Can you work these out from the model? Positions are in its coordinate system, mm. A direction names the side the tool comes from. Coordinates: 2 decimals unless noted, no trailing zeros. Loops run counter-clockwise (first coordinate to the right, second up) from the corner with the lowest first, then second, coordinate; pieces in that order, holes last. Notation, with made-up numbers: (75, 69) -> (94, 69) arc R8 cw to (94, 77) -> close; hole circle Ø5 at (-34.5, 65.25). An arc over 180 degrees is marked (long way). Use one line per item in the form item = value. Start each with the question number.
(1) I'm going to push flat-ended pins straight in: pin 1 (4 mm diameter, centred on x = -1, z = -2, fed in from -Y); pin 2 (3 mm diameter, centred on y = -8, z = -2.5, fed in from -X); pin 3 (6 mm diameter, centred on y = 2.5, z = 4, fed in from +X). Where does each tip first touch, or does it pass through?
(2) Imagine slicing it at B-B (x = 0). List the corners of the cut face in (y, z) for me, plus the area to 3 significant figures.
(3) I need wall thicknesses on line 1 (Y direction, x = -2.25, z = 3.25); line 2 (Z direction, x = 2, y = -13.5); line 3 (Z direction, x = -5, y = -8). Which ranges of each line are inside material? Lowest first, please. Write a range as [from, to].
(4) On a 3-axis mill with a long thin cutter (end or side, diameter ignored), from which of +Z, -Z, +X, -X, +Y, -Y can I reach the whole of each face in a straight line? I mean faces 1 (the conical face through (5.365, -8.619, 2.79)), 2 (the cylindrical face through (3.71, 3.45, 4.84)), 3 (the flat face through (0, 7, 0)). Say none if no direction works.
(5) Imagine slicing it at C-C (z = 0). List the corners of the cut face in (x, y) for me, plus the area to 3 significant figures.
(6) Imagine slicing it at A-A (y = -23). List the corners of the cut face in (x, z) for me.
```python
from build123d import *

# Parameters (mm, degrees)
SKETCH2_R           = 6.1
BOSS_EXTRUDE1_DEPTH = 7
SKETCH3_R           = 0.35
BOSS_EXTRUDE2_DEPTH = 9


with BuildPart() as part:
    # Sketch1 → Revolve1 (revolve)
    with BuildSketch(Plane.XY, mode=Mode.PRIVATE) as revolve1_sk:
        Polygon((0, 0), (6.25, 0), (5.85, -17), (0, -17), align=None)
    revolve(revolve1_sk.sketch.rotate(Axis((0, 0, 0), (0, -1, 0)), 90), axis=Axis((0, 0, 0), (0, -1, 0)))

    # Sketch2 → Boss-Extrude1 (add)
    with BuildSketch(Plane(origin=(0, 0, 0), x_dir=(1, 0, 0), z_dir=(0, 1, 0))):
        with Locations(Location((0, 0, 0), (0, 0, 90))):
            Circle(SKETCH2_R)
    extrude(amount=BOSS_EXTRUDE1_DEPTH)

    # Sketch3 → Boss-Extrude2 (add)
    with BuildSketch(Plane.XZ.offset(17)):
        with Locations(Location((-2.5, 0, 0), (0, 0, 90))):
            Circle(SKETCH3_R)
        with Locations(Location((2.5, 0, 0), (0, 0, 90))):
            Circle(SKETCH3_R)
    extrude(amount=BOSS_EXTRUDE2_DEPTH)


solid = part.part
```
Worked out:
q1.pin_1 = -17
q1.pin_2 = -5.98
q1.pin_3 = 6.02
q2.outline = (-17, -5.85) -> (0, -6.25) -> (0, -6.1) -> (7, -6.1) -> (7, 6.1) -> (0, 6.1) -> (0, 6.25) -> (-17, 5.85) -> close
q2.area = 291 mm2
q3.line_1 = [-17, 7]
q3.line_2 = [-5.59, 5.59]
q3.line_3 = [-3.43, 3.43]
q4.face_1 = -Y
q4.face_2 = +Y
q4.face_3 = +Z, -Z, +X, -X, +Y
q5.outline = (-6.25, 0) -> (-5.85, -17) -> (-2.85, -17) -> (-2.85, -26) -> (-2.15, -26) -> (-2.15, -17) -> (2.15, -17) -> (2.15, -26) -> (2.85, -26) -> (2.85, -17) -> (5.85, -17) -> (6.25, 0) -> (6.1, 0) -> (6.1, 7) -> (-6.1, 7) -> (-6.1, 0) -> close
q5.area = 304 mm2
q6.outline = circle Ø0.7 at (-2.5, 0); circle Ø0.7 at (2.5, 0)
